Can you work these out from the drawing? Everything is in mm from the part's minimum corner. Coordinates: 2 decimals unless noted, no trailing zeros. Loops run counter-clockwise (first coordinate to the right, second up) from the corner with the lowest first, then second, coordinate; pieces in that order, holes last.
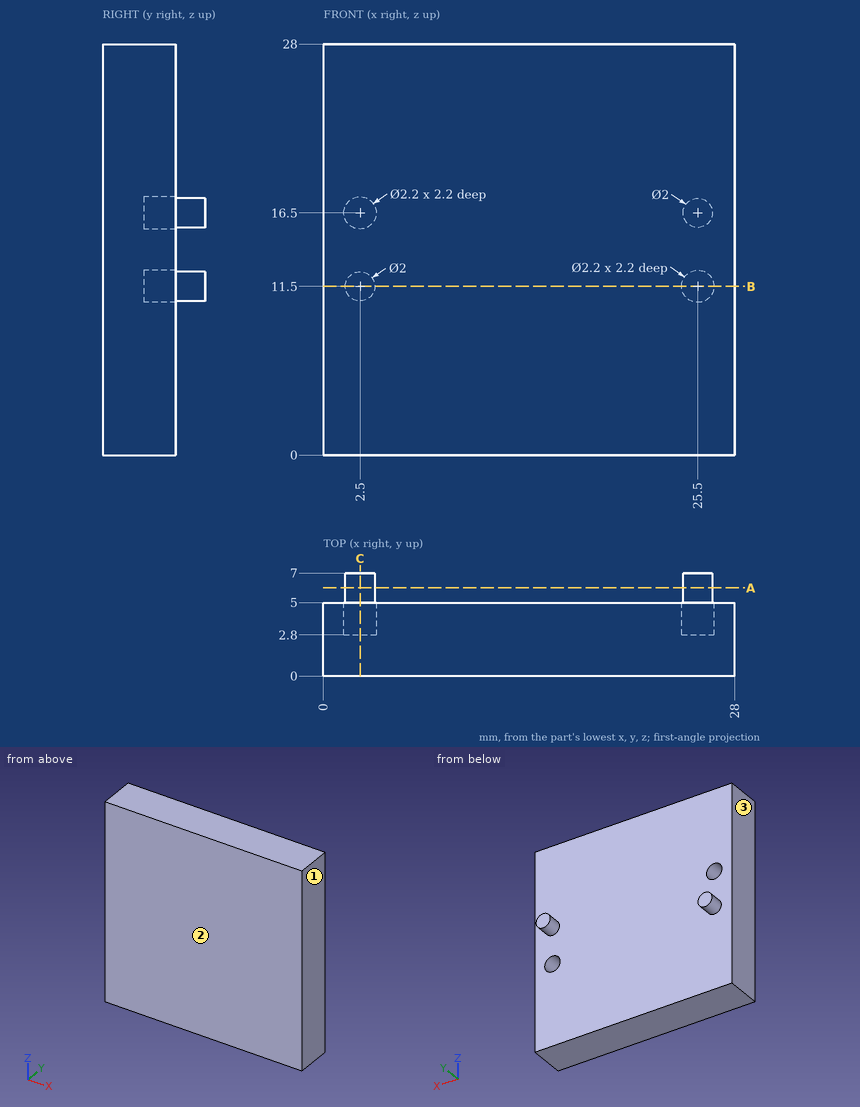
Item 1: Suppose I cut it at A-A, the plane y = 6. Please give me the cut outline in (x, z), plus the area to 3 significant figures.
Results are:
outline: circle Ø2 at (2.5, 11.5); circle Ø2 at (25.5, 16.5)
area: 6.28 mm2
Item 2: Suppose I cut it at B-B, the plane z = 11.5. Please give me the cut outline in (x, y).
Results are:
outline: (0, 0) - (28, 0) - (28, 5) - (26.6, 5) - (26.6, 2.8) - (24.4, 2.8) - (24.4, 5) - (3.5, 5) - (3.5, 7) - (1.5, 7) - (1.5, 5) - (0, 5) - close
Item 3: Suppose I cut it at C-C, the plane x = 2.5. Please give me the cut outline in (y, z).
Results are:
outline: (0, 0) - (5, 0) - (5, 10.5) - (7, 10.5) - (7, 12.5) - (5, 12.5) - (5, 15.4) - (2.8, 15.4) - (2.8, 17.6) - (5, 17.6) - (5, 28) - (0, 28) - close
Item 4: I need wall thicknesses on line 1 along Z through (x, y) = (25.5, 4.1); line 2 along Z through (x, y) = (2.5, 3.6); line 3 along Y through (x, z) = (26.25, 4). Which ranges of each line are inside material? Lowest first, please.
Results are:
line 1: z = 0 to 10.4, 12.6 to 28
line 2: z = 0 to 15.4, 17.6 to 28
line 3: y = 0 to 5
Item 5: I'm going to push flat-ended pins straight in: P1, Ø8, axis at x = 6.5, z = 5, coming from the +Y side; P2, Ø0.7, axis at x = 25, z = 11.5, coming from the +Y side; P3, Ø1.5, axis at x = 3.5, y = 6, coming from the -Z side. Where does each tip first touch, or does it pass through?
Results are:
P1: stops at y = 5
P2: stops at y = 2.8
P3: stops at z = 10.53
Item 6: We'd pull the mould along X, two halves only. Please class the marked faces 1, 2 and 3: +X half, -X half, draft (parallel to the pull), parting line (faces both ways), or undercut.
Results are:
face 1: +X half
face 2: draft
face 3: -X half
